from build123d import *

# Parameters (mm, degrees)
SKETCH2_W           = 25.4
SKETCH2_H           = 25.4
BOSS_EXTRUDE1_DEPTH = 254
SKETCH4_W           = 19.05
SKETCH4_H           = 19.05
CUT_EXTRUDE1_DEPTH  = 255.634208228
SKETCH5_R           = 3.2639
CUT_EXTRUDE2_DEPTH  = 304.8
SKETCH6_R           = 3.2639
CUT_EXTRUDE3_DEPTH  = 256.582569828
SKETCH8_R           = 3.2639
CUT_EXTRUDE4_DEPTH  = 256.582569828


with BuildPart() as part:
    # Sketch2 → Boss-Extrude1 (new body)
    with BuildSketch(Plane.XY):
        Rectangle(SKETCH2_W, SKETCH2_H)
    extrude(amount=BOSS_EXTRUDE1_DEPTH)

    # Sketch4 → Cut-Extrude1 (cut, through all)
    with BuildSketch(Plane.XY):
        Rectangle(SKETCH4_W, SKETCH4_H)
    extrude(amount=CUT_EXTRUDE1_DEPTH, mode=Mode.SUBTRACT)

    # Sketch5 → Cut-Extrude2 (cut)
    with BuildSketch(Plane(origin=(0, 12.7, 0), x_dir=(1, 0, 0), z_dir=(0, 1, 0))):
        with Locations(Location((0, -15.24, 0), (0, 0, 270))):
            Circle(SKETCH5_R)
    extrude(amount=-CUT_EXTRUDE2_DEPTH, mode=Mode.SUBTRACT)

    # Sketch6 → Cut-Extrude3 (cut, through all)
    with BuildSketch(Plane(origin=(0, 12.7, 0), x_dir=(1, 0, 0), z_dir=(0, 1, 0))):
        with Locations(Location((0, -247.65, 0), (0, 0, 270))):
            Circle(SKETCH6_R)
    extrude(amount=-CUT_EXTRUDE3_DEPTH, mode=Mode.SUBTRACT)

    # Sketch8 → Cut-Extrude4 (cut, through all)
    with BuildSketch(Plane(origin=(0, 12.7, 0), x_dir=(1, 0, 0), z_dir=(0, 1, 0))):
        with Locations(Location((0, -66.04, 0), (0, 0, 270))):
            Circle(SKETCH8_R)
        with Locations(Location((0, -40.64, 0), (0, 0, 270))):
            Circle(SKETCH8_R)
    extrude(amount=-CUT_EXTRUDE4_DEPTH, mode=Mode.SUBTRACT)


solid = part.part
The model under review builds one solid part; all positions refer to its coordinate system, in mm. A direction names the side the tool comes from. Give positions to 0.01 mm unless a question says otherwise; leave off trailing zeros. Order: outer loops, then holes, each group sorted by start corner. A loop starts at its lowest first (then second) coordinate and runs counter-clockwise, first axis right, second up. Notation, with made-up numbers: (20.25, 50) -> (24.25, 50) arc R24 cw to (24.25, 75) -> close; hole circle Ø1 at (45, -19.75). An arc over 180 degrees is marked (long way). Write item = value, one per line. Start each with the question number.
(1) For pin 1 Ø8 at (x, y) = (-2.5, -5) entering from +Z (1 decimal), flat-tipped, find the tip position at first contact; note if it passes through.
(2) Take a section at B-B (y = -0.5). Write out the cut boundary in (x, z) (3 decimals), plus the area to 3 significant figures.
(3) Take a section at A-A (z = 40.64). Write out the cut boundary in (x, y) (3 decimals).
(4) Draft analysis for pull direction X (two halves, no side actions). For faces 3 (the flat face through (11, 0, 254)), 4 (the flat face through (12.7, 0, 125)), 5 (the flat face through (-9.525, 0, 125)), 6 (the flat face through (9.525, 0, 125)), state which applies: +X half, -X half, draft (parallel to the pull), parting line (faces both ways), or undercut.
(5) Take a section at C-C (z = 184). Write out the cut boundary in (x, y) (3 decimals).
(6) Tool access review of faces 1 (the flat face through (0, -9.525, 125)), 2 (the cylindrical face through (0.14, -11.09, 62.78)): name each direction out of +Z, -Z, +X, -X, +Y, -Y from which nothing blocks a thin tool from reaching the whole face with its end or side.
(7) For L1, parallel to X at y = -11.35, z = 66.04; L2, parallel to X at y = 1.5, z = 195 (3 decimals), list the stretches that pass through material, from the lowest coordinate up. Write a range as from..to.
(8) Take a section at D-D (x = 0). State how many separate pieces and enclosed holes the cut face has, plus the area to 3 significant figures.
Returned:
q1.pin_1 = through
q2.outline = (-12.7, 0) -> (-9.525, 0) -> (-9.525, 254) -> (-12.7, 254) -> close; (9.525, 0) -> (12.7, 0) -> (12.7, 254) -> (9.525, 254) -> close
q2.area = 1,610 mm²
q3.outline = (-12.7, -12.7) -> (-3.264, -12.7) -> (-3.264, -9.525) -> (-9.525, -9.525) -> (-9.525, 9.525) -> (-3.264, 9.525) -> (-3.264, 12.7) -> (-12.7, 12.7) -> close; (3.264, -12.7) -> (12.7, -12.7) -> (12.7, 12.7) -> (3.264, 12.7) -> (3.264, 9.525) -> (9.525, 9.525) -> (9.525, -9.525) -> (3.264, -9.525) -> close
q4.face_3 = draft
q4.face_4 = +X half
q4.face_5 = undercut
q4.face_6 = undercut
q5.outline = (-12.7, -12.7) -> (12.7, -12.7) -> (12.7, 12.7) -> (-12.7, 12.7) -> close; hole (-9.525, -9.525) -> (9.525, -9.525) -> (9.525, 9.525) -> (-9.525, 9.525) -> close
q6.face_1 = +Z, -Z
q6.face_2 = +Y, -Y
q7.L1 = -12.7..-3.26, 3.26..12.7
q7.L2 = -12.7..-9.525, 9.525..12.7
q8.separate_pieces = 10
q8.enclosed_holes = 0
q8.area = 1,450 mm²
